from build123d import *

# Parameters (mm, degrees)
F1_DEPTH = 25
F2_T     = -2.5


with BuildPart() as f1:
    # F0 (on Front) → F1 (new body)
    with BuildSketch(Plane.XZ):
        Polygon((10, 40), (-10, 40), (-10, 0), (-211.1074434719, 0), (-211.1074434719, -25.2444452331), (185.367203297, -25.2444452331), (185.367203297, 0), (10, 0), align=None)
    extrude(amount=F1_DEPTH)

    # F2
    f2_openings = [f1.faces().sort_by_distance(p)[0] for p in [
        (-11.917552, -25, -10.207725),
    ]]
    offset(amount=F2_T, openings=f2_openings, kind=Kind.INTERSECTION)


solid = f1.part
The listing builds one solid part. Answer for the finished solid, in the listing's coordinates (mm). A direction names the side the tool comes from. Give positions to 0.01 mm unless a question says otherwise; leave off trailing zeros. Order: outer loops, then holes, each group sorted by start corner. A loop starts at its lowest first (then second) coordinate and runs counter-clockwise, first axis right, second up. Notation, with made-up numbers: (88, -1.5) - (145, -1.5) arc R6 cw to (145, 2.5) - close; hole circle Ø9 at (26, -34.75). An arc over 180 degrees is marked (long way). Answer as CSV lines item,"result".
Q1. A cutting plane is placed at C-C, the plane z = 31.5. Determine the outline of the cut face in (x, y).
Answer key:
outline,"(-10, -25) - (-7.5, -25) - (-7.5, -2.5) - (7.5, -2.5) - (7.5, -25) - (10, -25) - (10, 0) - (-10, 0) - close"
Q2. Each of these flat-tipped pins is pushed along its axis until it touches: pin 1 Ø7.5 at (y, z) = (-8, 18.5) entering from +X; pin 2 Ø11 at (y, z) = (-11, 22) entering from -X; pin 3 Ø5 at (x, y) = (-71.5, -15) entering from +Z. Where does it stop, or does it pass through?
Answer key:
pin 1,"stops at x = 10"
pin 2,"stops at x = -10"
pin 3,"stops at z = 0"
Q3. A cutting plane is placed at A-A, the plane x = 65.5. Determine the outline of the cut face in (y, z), and give its area (3 significant figures).
Answer key:
outline,"(-25, -25.24) - (0, -25.24) - (0, 0) - (-25, 0) - (-25, -2.5) - (-2.5, -2.5) - (-2.5, -22.74) - (-25, -22.74) - close"
area,"176 mm^2"
Q4. Determine the mould class of faces 5 (the face through (-208.607, -14, -12)), 6 (the face through (-10, -12, 20)), 7 (the face through (185.367, -12, -13)), 8 (the face through (0, -12, 40)) for opening direction X: pulls with the +X half, pulls with the -X half, needs draft (parallel to the pull), parting line crosses it, or undercut.
Answer key:
face 5,"undercut"
face 6,"pulls with the -X half"
face 7,"pulls with the +X half"
face 8,"needs draft"
Q5. Which of the six approach directions +Z, -Z, +X, -X, +Y, -Y give full straight-line access (tool end or side, diameter ignored) to faces 1 (the face through (-211.107, -12, -12)), 2 (the face through (-109, -12, 0)), 3 (the face through (99, -12, 0)), 4 (the face through (7.5, -14, 17))?
Answer key:
face 1,"+Z, -Z, -X, +Y, -Y"
face 2,"+Z, -X, +Y, -Y"
face 3,"+Z, +X, +Y, -Y"
face 4,"-Y"
Q6. Straight lines are drawn through the part: L1, parallel to Z at x = -149.5, y = -3.75; L2, parallel to X at y = -7.75, z = -6; L3, parallel to Z at x = 9, y = -19.75. For each, find the intervals that lie inside material, in ascending order.
Answer key:
L1,"z = -25.24 to -22.74, -2.5 to 0"
L2,"x = -211.11 to -208.61, 182.87 to 185.37"
L3,"z = -25.24 to -22.74, -2.5 to 40"
Q7. A cutting plane is placed at B-B, the plane y = -15.75. Determine the outline of the cut face in (x, z).
Answer key:
outline,"(-211.11, -25.24) - (185.37, -25.24) - (185.37, 0) - (10, 0) - (10, 40) - (-10, 40) - (-10, 0) - (-211.11, 0) - close; hole (-208.61, -22.74) - (182.87, -22.74) - (182.87, -2.5) - (7.5, -2.5) - (7.5, 37.5) - (-7.5, 37.5) - (-7.5, -2.5) - (-208.61, -2.5) - close"
